Verification items for the finished model (mm, model axes). A direction names the side the tool comes from. Round coordinates to 2 decimals unless told otherwise and drop trailing zeros. Order: outer loops, then holes, each group sorted by start corner. A loop starts at its lowest first (then second) coordinate and runs counter-clockwise, first axis right, second up. Notation, with made-up numbers: M -28.75,37 L 5.25,37 A33 cw 5.25,71 Z; hole C 25.25,27 d8. An arc over 180 degrees is marked long. One line per item, written item: value. Start each with the question number.
from build123d import *

# Parameters (mm, degrees)
F0_R     = 6.85
F1_DEPTH = 0.9
F2_R     = 4.2
F3_DEPTH = 1.2
F5_DEPTH = 2.1
F6_SIZE  = 0.3


with BuildPart() as f1:
    # F0 (on Top) → F1 (new body)
    with BuildSketch(Plane.XY):
        Circle(F0_R)
    extrude(amount=F1_DEPTH)

    # F2 (on face) → F3 (join)
    with BuildSketch(Plane.XY.offset(0.9)):
        Circle(F2_R)
    extrude(amount=F3_DEPTH)

    # F4 (on face) → F5 (cut, through all)
    with BuildSketch(Plane.XY.offset(2.1)):
        with BuildLine():
            ThreePointArc((-1.65, -2.5651510677), (1.4611639196, -2.677218706), (3.05, 0))
            ThreePointArc((3.05, 0), (1.4611639196, 2.677218706), (-1.65, 2.5651510677))
            Line((-1.65, 2.5651510677), (-1.65, -2.5651510677))
        make_face()
    extrude(amount=-F5_DEPTH, mode=Mode.SUBTRACT)

    # F6
    f6_edges = [f1.edges().sort_by_distance(p)[0] for p in [
        (-6.85, 0, 0),
        (3.05, 0, 0),
        (-1.65, 0, 0),
    ]]
    chamfer(f6_edges, length=F6_SIZE)


solid = f1.part
1. Depth check by flat-ended pin: pin 1 (0.9 mm diameter, centred on y = -1, z = 1.5, fed in from +X); pin 2 (2 mm diameter, centred on x = 3, y = -4, fed in from -Z). Enter the tip coordinate at first touch or a pass-through.
2. Section check B-B (z = 1.5). Record the cut outline in (x, y), and give its area (3 significant figures).
3. Draft check along X on faces 1 (the face through (-1.65, 0, 1)), 2 (the face through (-2, 0, 2.1)), 3 (the face through (4.006, 1.262, 1.492)). Enter one of: released by +X, released by -X, zero draft, split by the parting line, or undercut.
4. Scan lines: line 1 along Y through (x, z) = (0, 0.5); line 2 along Z through (x, y) = (-4.5, -3); line 3 along X through (y, z) = (-1.5, 0.85). Record each from-to range of solid material in increasing order.
5. Section check A-A (x = 0). Record the cut outline in (y, z).
6. Tool access check on faces 4 (the face through (-3, 0, 0)), 5 (the face through (-0.1, -4.5, 0.9)). Record the directions out of +Z, -Z, +X, -X, +Y, -Y that give a thin tool (end or side, any length) a straight path to the whole face; none if there is none.
Geometry check:
1. pin 1: stops at x = 4.16
1. pin 2: stops at z = 0
2. outline: C 0,0 d8.4; hole M -1.65,-2.57 A3.05 ccw long -1.65,2.57 Z
2. area: 31.3 mm²
3. face 1: undercut
3. face 2: zero draft
3. face 3: split by the parting line
4. line 1: y = -6.85 to -3.05, 3.05 to 6.85
4. line 2: z = 0 to 0.9
4. line 3: x = -6.68 to -1.65, 2.66 to 6.68
5. outline: M -6.85,0.3 L -6.55,0 L -3.35,0 L -3.05,0.3 L -3.05,2.1 L -4.2,2.1 L -4.2,0.9 L -6.85,0.9 Z; M 3.05,0.3 L 3.35,0 L 6.55,0 L 6.85,0.3 L 6.85,0.9 L 4.2,0.9 L 4.2,2.1 L 3.05,2.1 Z
6. face 4: -Z, +X, -X, +Y, -Y
6. face 5: +Z
